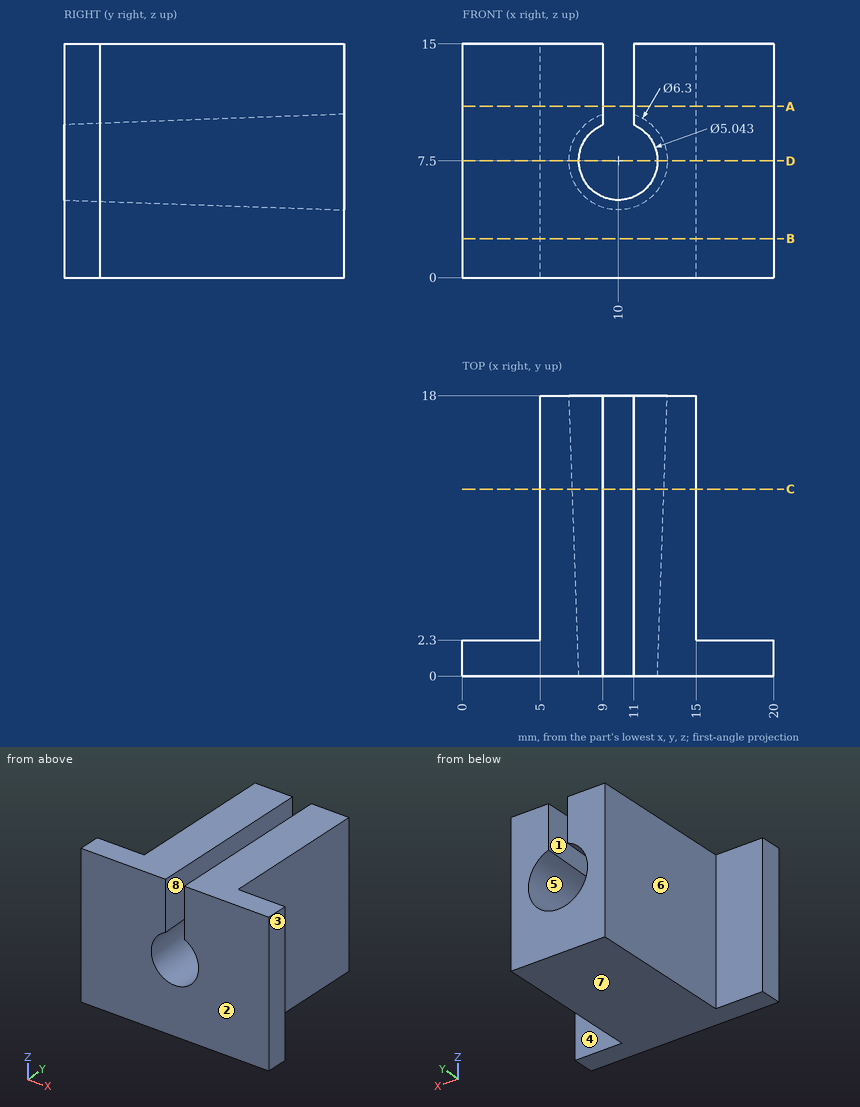
Geometry check sheet. Reference: drawing and pictorial views, mm from the part's lowest x, y, z. A direction names the side the tool comes from. Give positions to 0.01 mm unless a question says otherwise; leave off trailing zeros. Loops run counter-clockwise (first coordinate to the right, second up) from the corner with the lowest first, then second, coordinate; pieces in that order, holes last. Notation, with made-up numbers: M 49.25,45.5 L 58.25,45.5 A16 ccw 58.25,60.5 Z; hole C 62.25,34 d6. An arc over 180 degrees is marked long. Use a Markdown table: item, result. Add a question column.
Q1. Mould release check, pull along X, two halves, no side actions. Record for the marked faces 1, 2 and 3: pulls with the +X half, pulls with the -X half, needs draft (parallel to the pull), parting line crosses it, or undercut.
Q2. Tool access check on the marked faces 4, 5, 6, 7 and 8. Record the directions out of +Z, -Z, +X, -X, +Y, -Y that give a thin tool (end or side, any length) a straight path to the whole face; none if there is none.
Q3. Scan lines: line 1 along X through (y, z) = (13.25, 12); line 2 along X through (y, z) = (14, 4.75) (1 decimal); line 3 along Y through (x, z) = (2.75, 6.75). Record each from-to range of solid material in increasing order. Write a range as [from, to].
Q4. Go/stop test with flat-tipped pins: pin 1 (2.5 mm diameter, centred on y = 7.5, z = 13.5, fed in from +X); pin 2 (1.5 mm diameter, centred on x = 11.5, y = 16, fed in from -Z); pin 3 (1 mm diameter, centred on y = 16, z = 2.5, fed in from -X). Record where each tip stops, or that it passes through.
Q5. Sectioned sample at A-A, the plane z = 11. Record the cut outline in (x, y).
Q6. Sectioned sample at D-D, the plane z = 7.5. Record the cut outline in (x, y), then the cut area to 3 significant figures.
Q7. Sectioned sample at C-C, the plane y = 12. Record the cut outline in (x, z) (1 decimal), then the cut area to 3 significant figures.
Q8. Sectioned sample at B-B, the plane z = 2.5. Record the cut outline in (x, y), then the cut area to 3 significant figures.
Verdict:
| question | item | result |
|---|---|---|
| 1 | face 1 | undercut |
| 1 | face 2 | needs draft |
| 1 | face 3 | pulls with the +X half |
| 2 | face 4 | +Z, -Z, +X, +Y |
| 2 | face 5 | +Y |
| 2 | face 6 | +Z, -Z, -X, +Y |
| 2 | face 7 | -Z, +X, -X, +Y, -Y |
| 2 | face 8 | +Z, +Y, -Y |
| 3 | line 1 | [5, 9], [11, 15] |
| 3 | line 2 | [5, 8.8], [11.2, 15] |
| 3 | line 3 | [0, 2.3] |
| 4 | pin 1 | x = 15 |
| 4 | pin 2 | z = 0 |
| 4 | pin 3 | x = 5 |
| 5 | outline | M 0,0 L 9,0 L 9,18 L 5,18 L 5,2.3 L 0,2.3 Z; M 11,0 L 20,0 L 20,2.3 L 15,2.3 L 15,18 L 11,18 Z |
| 6 | outline | M 0,0 L 7.48,0 L 6.85,18 L 5,18 L 5,2.3 L 0,2.3 Z; M 12.52,0 L 20,0 L 20,2.3 L 15,2.3 L 15,18 L 13.15,18 Z |
| 6 | area | 101 mm^2 |
| 7 | outline | M 5,0 L 15,0 L 15,15 L 11,15 L 11,10.3 A2.9 cw long 9,10.3 L 9,15 L 5,15 Z |
| 7 | area | 114 mm^2 |
| 8 | outline | M 0,0 L 20,0 L 20,2.3 L 15,2.3 L 15,18 L 5,18 L 5,2.3 L 0,2.3 Z |
| 8 | area | 203 mm^2 |
